```python
from build123d import *

# Parameters (mm, degrees)
F1_DEPTH = 22
F3_DEPTH = 2.3
F4_R     = 3.675
F4_R_2   = 2.3
F5_DEPTH = 1.45
F6_R     = 0.85
F7_DEPTH = 25


# Not quite as in the source:
# - a fillet or chamfer that OpenCascade refuses, or shapes differently, is made with other operations: its cross-section is extruded or revolved along the edge and cut away or added


with BuildPart() as f1:
    # F0 (on Front) → F1 (new body)
    with BuildSketch(Plane.XZ):
        Polygon((-36.1197131506, 22.3681449045), (-39.6497131506, 22.3681449045), (-39.6497131506, 18.8381449045), (-40.5097131506, 18.8381449045), (-40.5097131506, 17.6681449045), (-39.6497131506, 17.6681449045), (-36.1197131506, 17.6681449045), (-35.2597131506, 17.6681449045), (-35.2597131506, 18.8381449045), (-36.1197131506, 18.8381449045), align=None)
    extrude(amount=F1_DEPTH)

    # F2 (on face) → F3 (join)
    with BuildSketch(Plane.XY.offset(22.3681449045)):
        with BuildLine():
            Line((-36.1197131506, -12.4747118363), (-36.1197131506, -9.5252881637))
            ThreePointArc((-36.1197131506, -9.5252881637), (-37.8847131506, -8.7), (-39.6497131506, -9.5252881637))
            Line((-39.6497131506, -9.5252881637), (-39.6497131506, -12.4747118363))
            ThreePointArc((-39.6497131506, -12.4747118363), (-37.8847131506, -13.3), (-36.1197131506, -12.4747118363))
        make_face()
        with BuildLine():
            Line((-39.6497131506, -12.4747118363), (-39.6497131506, -9.5252881637))
            ThreePointArc((-39.6497131506, -9.5252881637), (-40.1847131506, -11), (-39.6497131506, -12.4747118363))
        make_face()
        with BuildLine():
            ThreePointArc((-36.1197131506, -12.4747118363), (-35.7225961325, -11.7843787351), (-35.5847131506, -11))
            ThreePointArc((-35.5847131506, -11), (-35.7225961325, -10.2156212649), (-36.1197131506, -9.5252881637))
            Line((-36.1197131506, -9.5252881637), (-36.1197131506, -12.4747118363))
        make_face()
    extrude(amount=F3_DEPTH)

    # F4 (on face) → F5 (join)
    with BuildSketch(Plane.XY.offset(24.6681449045)):
        with Locations((-37.8847131506, -11)):
            Circle(F4_R)
        with Locations((-37.8847131506, -11)):
            Circle(F4_R_2, mode=Mode.SUBTRACT)
        with Locations((-37.8847131506, -11)):
            Circle(F4_R_2)
    extrude(amount=F5_DEPTH)

    # F6 (on face) → F7 (cut)
    with BuildSketch(Plane(origin=(0, 0, 17.6681449045), x_dir=(1, 0, 0), z_dir=(0, 0, -1))):
        with Locations((-37.8847131506, 18)):
            Circle(F6_R)
        with Locations((-37.8847131506, 4)):
            Circle(F6_R)
    extrude(amount=-F7_DEPTH, mode=Mode.SUBTRACT)

    # F8: chamfer of 2 on 1 edges, made by hand

    # F8_s1 → F8_t2 (revolve, cut)
    with BuildSketch(Plane.XZ.offset(18)):
        Polygon((-35.0347131506, 22.3681449045), (-37.0347131506, 20.3681449045), (-37.0347131506, 22.3681449045), align=None)
    revolve(axis=Axis((-37.8847131506, -18, 22.3681449045), (0, 0, -1)), mode=Mode.SUBTRACT)

    # F9: chamfer of 2 on 1 edges, made by hand

    # F9_s1 → F9_t2 (revolve, cut)
    with BuildSketch(Plane.XZ.offset(4)):
        Polygon((-35.0347131506, 22.3681449045), (-37.0347131506, 20.3681449045), (-37.0347131506, 22.3681449045), align=None)
    revolve(axis=Axis((-37.8847131506, -4, 22.3681449045), (0, 0, -1)), mode=Mode.SUBTRACT)


solid = f1.part
```
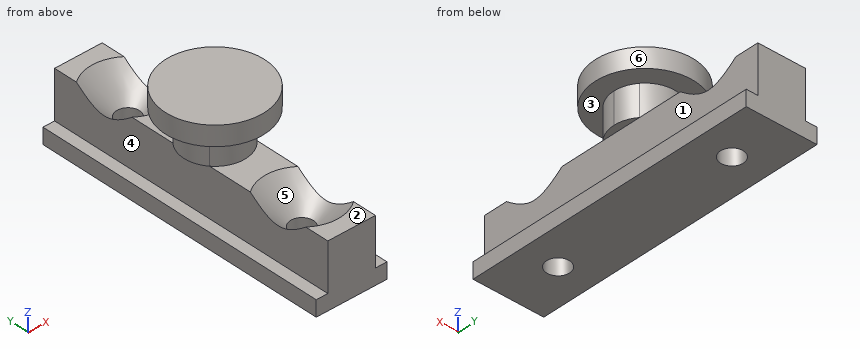
CAD build for the part. Positions are in the model's coordinates, mm. Face numbers are marked on the shaded views. A direction names the side the tool comes from. Round coordinates to 2 decimals unless told otherwise and drop trailing zeros. Write each loop counter-clockwise with the first axis right and the second up, starting at its lowest first coordinate (ties: lowest second). Pieces come first, ordered by that corner, then holes.
Item 1: Drill centre lines: L1, parallel to X at y = -18, z = 18.4; L2, parallel to Y at x = -38, z = 19.75; L3, parallel to X at y = -18, z = 19.8. Where is each one in solid material? Low to high.
Filled in:
L1: x = -40.51 to -38.73, -37.03 to -35.26
L2: y = -22 to -18.84, -17.16 to -4.84, -3.16 to 0
L3: x = -39.65 to -38.73, -37.03 to -36.12
Item 2: Band-saw the part on C-C on x = -35. Write the cut outline in (y, z), then the cut area to 3 significant figures.
Filled in:
outline: (-13.28, 24.67) - (-8.72, 24.67) - (-8.72, 26.12) - (-13.28, 26.12) - close
area: 6.60 mm2
Item 3: Mould opens along X. For the marked faces 4, 5 and 6 say: released by +X, released by -X, zero draft, split by the parting line, or undercut.
Filled in:
face 4: released by -X
face 5: undercut
face 6: split by the parting line
Item 4: Tool access for the marked faces 1, 2 and 3: list every direction of +Z, -Z, +X, -X, +Y, -Y with a clear straight run to the whole face (end or side of a thin tool).
Filled in:
face 1: +X, +Y, -Y
face 2: +Z, +X, -X, -Y
face 3: none
Item 5: Band-saw the part on A-A on y = -18. Write the cut outline in (x, z), then the cut area to 3 significant figures.
Filled in:
outline: (-40.51, 17.67) - (-38.73, 17.67) - (-38.73, 20.37) - (-39.65, 21.28) - (-39.65, 18.84) - (-40.51, 18.84) - close; (-37.03, 17.67) - (-35.26, 17.67) - (-35.26, 18.84) - (-36.12, 18.84) - (-36.12, 21.28) - (-37.03, 20.37) - close
area: 7.79 mm2
Item 6: Band-saw the part on D-D on z = 25. Write the cut outline in (x, y) (3 decimals), then the cut area to 3 significant figures.
Filled in:
outline: circle Ø7.35 at (-37.885, -11)
area: 42.4 mm2
Item 7: Drop flat-ended pins along their axis: pin 1 Ø1.5 at (y, z) = (-9, 21) entering from -X; pin 2 Ø0.6 at (y, z) = (-10, 18.5) entering from +X; pin 3 Ø1.5 at (x, z) = (-40, 18.5) entering from +Y; pin 4 Ø0.9 at (x, y) = (-40, -5.5) entering from +Z. Give the stop position or say it passes through.
Filled in:
pin 1: stops at x = -39.65
pin 2: stops at x = -35.26
pin 3: stops at y = 0
pin 4: stops at z = 22.03
Item 8: Band-saw the part on B-B on z = 23.75. Write the cut outline in (x, y).
Filled in:
outline: circle Ø4.6 at (-37.88, -11)
